```python
from build123d import *

# Parameters (mm, degrees)
SKETCH2_W           = 25
SKETCH2_H           = 25
BOSS_EXTRUDE1_DEPTH = 25
FILLET2_R           = 10
FILLET3_R           = 10
CUT_EXTRUDE1_START  = -5
SKETCH3_W           = 8
SKETCH3_H           = 8
SKETCH3_W_2         = 6
SKETCH3_H_2         = 6
CUT_EXTRUDE1_DEPTH  = 5
FILLET5_R           = 5
CUT_EXTRUDE2_DEPTH  = 5
FILLET6_R           = 4
SKETCH6_R           = 1.5
CUT_EXTRUDE3_DEPTH  = 15
CUT_EXTRUDE4_DEPTH  = 5


with BuildPart() as part:
    # Sketch2 → Boss-Extrude1 (new body)
    with BuildSketch(Plane(origin=(0, 0, 0), x_dir=(1, 0, 0), z_dir=(0, 1, 0))):
        Rectangle(SKETCH2_W, SKETCH2_H)
    extrude(amount=BOSS_EXTRUDE1_DEPTH)

    # Fillet2
    fillet2_edges = [part.edges().sort_by_distance(p)[0] for p in [
        (12.5, 12.5, 12.5),
        (-12.5, 12.5, 12.5),
    ]]
    fillet(fillet2_edges, radius=FILLET2_R)

    # Fillet3
    fillet3_edges = [part.edges().sort_by_distance(p)[0] for p in [
        (0, 25, 12.5),
        (12.5, 25, -5),
        (9.571067812, 25, 9.571067812),
        (-9.571067812, 25, 9.571067812),
        (-12.5, 25, -5),
    ]]
    fillet(fillet3_edges, radius=FILLET3_R)

    # Sketch3 → Cut-Extrude1 (cut)
    # profile 1 of 2: a face of its own
    with BuildSketch(Plane.XZ.offset(CUT_EXTRUDE1_START)):
        with BuildLine():
            ThreePointArc((12.5, 2.5), (9.571067812, 9.571067812), (2.5, 12.5))
            Line((2.5, 12.5), (-2.5, 12.5))
            ThreePointArc((-2.5, 12.5), (-9.571067812, 9.571067812), (-12.5, 2.5))
            Line((-12.5, 2.5), (-12.5, -12.5))
            Line((-12.5, -12.5), (12.5, -12.5))
            Line((12.5, -12.5), (12.5, 2.5))
        make_face()
        Rectangle(SKETCH3_W, SKETCH3_H, mode=Mode.SUBTRACT)
    # profile 2 of 2: a face of its own
    with BuildSketch(Plane.XZ.offset(CUT_EXTRUDE1_START)):
        Rectangle(SKETCH3_W_2, SKETCH3_H_2)
    extrude(amount=CUT_EXTRUDE1_DEPTH, mode=Mode.SUBTRACT)

    # Fillet5
    fillet5_edges = [part.edges().sort_by_distance(p)[0] for p in [
        (9.571067812, 5, 9.571067812),
        (12.5, 5, -5),
        (-12.5, 5, -5),
        (-9.571067812, 5, 9.571067812),
        (0, 5, 12.5),
    ]]
    fillet(fillet5_edges, radius=FILLET5_R)

    # Sketch5 → Cut-Extrude2 (cut)
    with BuildSketch(Plane.XZ):
        Polygon((-3, 3), (-3, 4.768124317), (3, 4.768124317), (3, -4.905831879), (-3, -4.905831879), align=None)
    extrude(amount=-CUT_EXTRUDE2_DEPTH, mode=Mode.SUBTRACT)

    # Fillet6
    fillet6_edges = [part.edges().sort_by_distance(p)[0] for p in [
        (3.5, 0, -4),
        (3.5, 0, 4),
        (-3.5, 0, -4),
        (-3.5, 0, 4),
    ]]
    fillet(fillet6_edges, radius=FILLET6_R - 0.0001)  # a hair under: the kernel refuses the full size

    # Sketch6 → Cut-Extrude3 (cut)
    with BuildSketch(Plane.ZY.offset(4)):
        with Locations((0, 3)):
            Circle(SKETCH6_R)
    extrude(amount=-CUT_EXTRUDE3_DEPTH, mode=Mode.SUBTRACT)

    # Sketch7 → Cut-Extrude4 (cut)
    with BuildSketch(Plane(origin=(0, 0, -12.5), x_dir=(-1, 0, 0), z_dir=(0, 0, -1))):
        with BuildLine():
            Line((-12.5, 15), (-12.5, 10))
            ThreePointArc((-12.5, 10), (-11.035533906, 6.464466094), (-7.5, 5))
            Line((-7.5, 5), (7.5, 5))
            ThreePointArc((7.5, 5), (11.035533906, 6.464466094), (12.5, 10))
            Line((12.5, 10), (12.5, 15))
            ThreePointArc((12.5, 15), (9.571067812, 22.071067812), (2.5, 25))
            Line((2.5, 25), (-2.5, 25))
            ThreePointArc((-2.5, 25), (-9.571067812, 22.071067812), (-12.5, 15))
        make_face()
    extrude(amount=-CUT_EXTRUDE4_DEPTH, mode=Mode.SUBTRACT)


solid = part.part
```
The listing builds one solid part. Answer for the finished solid, in the listing's coordinates (mm). A direction names the side the tool comes from. Give positions to 0.01 mm unless a question says otherwise; leave off trailing zeros. Order: outer loops, then holes, each group sorted by start corner. A loop starts at its lowest first (then second) coordinate and runs counter-clockwise, first axis right, second up. Notation, with made-up numbers: (-13, 68.25) -> (21, 68.25) arc R20 ccw to (21, 102.25) -> close; hole circle Ø8 at (67, -23.75). An arc over 180 degrees is marked (long way). One line per item, written item: value.
1) Determine the mould class of faces 5 (the flat face through (4, 1, 0)), 6 (the cylindrical face through (3.507, 1.141, -2.797)), 7 (the cylindrical face through (-3.507, 1.536, -0.325)) for opening direction Y: pulls with the +Y half, pulls with the -Y half, needs draft (parallel to the pull), parting line crosses it, or undercut.
Reported:
face 5: needs draft
face 6: pulls with the -Y half
face 7: undercut
2) Flat-ended cylindrical pins translate along their axes: P1, Ø6, axis at x = -1, y = 22.5, coming from the +Z side; P2, Ø6, axis at x = 9.5, y = 8.5, coming from the +Z side; P3, Ø8, axis at x = 3.5, z = 0.5, coming from the +Y side; P4, Ø1.5, axis at y = 10, z = 4.5, coming from the -X side. Find the tip coordinate at first contact, or state that the pin passes through.
Reported:
P1: stops at z = 11.43
P2: stops at z = 11.56
P3: stops at y = 25
P4: stops at x = -12.42
3) Find section A-A, the plane y = 2.25. Determine the outline of the cut face in (x, z).
Reported:
outline: (-4, -3.6) -> (-3, -3.6) -> (-3, -1.3) -> (-4, -1.3) -> close; (-4, 1.3) -> (-3, 1.3) -> (-3, 3.6) -> (-4, 3.6) -> close; (3, -3.6) -> (4, -3.6) -> (4, -1.3) -> (3, -1.3) -> close; (3, 1.3) -> (4, 1.3) -> (4, 3.6) -> (3, 3.6) -> close
4) Find section B-B, the plane z = -4.5. Determine the outline of the cut face in (x, y).
Reported:
outline: (-12.5, 10) arc R5 ccw to (-7.5, 5) -> (7.5, 5) arc R5 ccw to (12.5, 10) -> (12.5, 15) arc R10 ccw to (2.5, 25) -> (-2.5, 25) arc R10 ccw to (-12.5, 15) -> close
5) Find the intervals of material crossed by line 1 (Y direction, x = -3.65, z = 0); line 2 (Y direction, x = -2, z = -3.75); line 3 (Z direction, x = -3.25, y = 3.5), in increasing order.
Reported:
line 1: y = 0 to 1.5, 4.5 to 24.93
line 2: y = 5 to 25
line 3: z = -3.97 to -1.41, 1.41 to 3.97
6) Find section D-D, the plane y = 19.5. Determine the outline of the cut face in (x, z).
Reported:
outline: (-11.43, -7.5) -> (11.43, -7.5) -> (11.43, 2.5) arc R8.93 ccw to (2.5, 11.43) -> (-2.5, 11.43) arc R8.93 ccw to (-11.43, 2.5) -> close
7) A tool of negligible diameter and unlimited length cuts with its end or side. For faces 1 (the flat face through (-3, 1, 0)), 2 (the flat face through (0, 25, -3)), 3 (the flat face through (-3.5, 4.5, -4)), 4 (the flat face through (-3.5, 4.5, 4)), from which of +Z, -Z, +X, -X, +Y, -Y can it reach the whole face along a straight path? Write none if from no direction.
Reported:
face 1: +Z, -Z, -Y
face 2: +Z, -Z, +X, -X, +Y
face 3: -Z, +X, -X, -Y
face 4: +Z, +X, -X, -Y
8) Find section C-C, the plane x = -1.25. Determine the outline of the cut face in (y, z).
Reported:
outline: (5, -7.5) -> (25, -7.5) -> (25, 2.5) arc R10 ccw to (15, 12.5) -> (10, 12.5) arc R5 ccw to (5, 7.5) -> close
